Input: part model. Units: mm. Frame: model coordinates. Round coordinates to 2 decimals unless told otherwise and drop trailing zeros. Loops run counter-clockwise (first coordinate to the right, second up) from the corner with the lowest first, then second, coordinate; pieces in that order, holes last. Notation, with made-up numbers: (-37.5, -31) -> (-13.5, -31) arc R16 cw to (-13.5, -19) -> close; hole circle Ø4 at (10.25, 42.5). An arc over 180 degrees is marked (long way). Answer as a JSON object with one key per item and string values.
```python
from build123d import *

# Parameters (mm, degrees)
SKETCH1_W           = 170
SKETCH1_H           = 120
SKETCH1_R           = 2.5
BOSS_EXTRUDE1_DEPTH = 3
CUT_EXTRUDE1_REACH  = 106.087
SKETCH2_R           = 12.5


with BuildPart() as part:
    # Sketch1 → Boss-Extrude1 (new body)
    with BuildSketch(Plane(origin=(0, 0, 0), x_dir=(1, 0, 0), z_dir=(0, 1, 0))):
        Rectangle(SKETCH1_W, SKETCH1_H)
        with Locations(Location((-65, 47, 0), (0, 0, 270))):
            Circle(SKETCH1_R, mode=Mode.SUBTRACT)
        with Locations(Location((-65, -47, 0), (0, 0, 90))):
            Circle(SKETCH1_R, mode=Mode.SUBTRACT)
        with Locations(Location((65, -47, 0), (0, 0, 270))):
            Circle(SKETCH1_R, mode=Mode.SUBTRACT)
        with Locations(Location((65, 47, 0), (0, 0, 90))):
            Circle(SKETCH1_R, mode=Mode.SUBTRACT)
    extrude(amount=BOSS_EXTRUDE1_DEPTH)

    # Sketch2 → Cut-Extrude1 (cut, up to next)
    with BuildSketch(Plane(origin=(0, 3, 0), x_dir=(1, 0, 0), z_dir=(0, 1, 0)), mode=Mode.PRIVATE) as cut_extrude1_sk1:
        with Locations((-85, -20)):
            Circle(SKETCH2_R)
    cut_extrude1_tool1 = extrude(cut_extrude1_sk1.sketch, amount=-CUT_EXTRUDE1_REACH, mode=Mode.PRIVATE) & part.part
    add(cut_extrude1_tool1.solids().sort_by_distance((-85, 3, 20))[0], mode=Mode.SUBTRACT)


solid = part.part
```
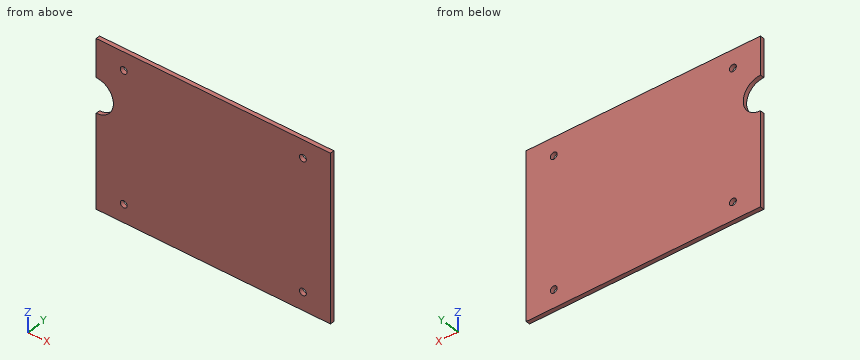
1) Section A-A, the plane z = 47. Output: boundary loops of the cut face in (x, y), plus the area to 3 significant figures.
Output:
{"outline": "(-85, 0) -> (-67.5, 0) -> (-67.5, 3) -> (-85, 3) -> close; (-62.5, 0) -> (62.5, 0) -> (62.5, 3) -> (-62.5, 3) -> close; (67.5, 0) -> (85, 0) -> (85, 3) -> (67.5, 3) -> close", "area": "480 mm^2"}
2) Section B-B, the plane x = 65. Output: boundary loops of the cut face in (y, z), plus the area to 3 significant figures.
Output:
{"outline": "(0, -60) -> (3, -60) -> (3, -49.5) -> (0, -49.5) -> close; (0, -44.5) -> (3, -44.5) -> (3, 44.5) -> (0, 44.5) -> close; (0, 49.5) -> (3, 49.5) -> (3, 60) -> (0, 60) -> close", "area": "330 mm^2"}
3) Section D-D, the plane z = 20. Output: boundary loops of the cut face in (x, y), plus the area to 4 significant figures.
Output:
{"outline": "(-72.5, 0) -> (85, 0) -> (85, 3) -> (-72.5, 3) -> close", "area": "472.5 mm^2"}
4) Section C-C, the plane y = 1.2. Output: boundary loops of the cut face in (x, z).
Output:
{"outline": "(-85, -60) -> (85, -60) -> (85, 60) -> (-85, 60) -> (-85, 32.5) arc R12.5 cw to (-85, 7.5) -> close; hole circle Ø5 at (-65, -47); hole circle Ø5 at (-65, 47); hole circle Ø5 at (65, -47); hole circle Ø5 at (65, 47)"}
5) Ray query, probe 1 along X at (y, z) = (2.4, 47); probe 2 along X at (y, z) = (1.35, 46); probe 3 along X at (y, z) = (1.1, 11). Return the intervals inside material, ascending.
Output:
{"probe 1": "x = -85 to -67.5, -62.5 to 62.5, 67.5 to 85", "probe 2": "x = -85 to -67.29, -62.71 to 62.71, 67.29 to 85", "probe 3": "x = -76.33 to 85"}
